Build history of the part. All positions in model axes, mm. Face numbers are marked on the shaded views. Round coordinates to 2 decimals unless told otherwise and drop trailing zeros. Write each loop counter-clockwise with the first axis right and the second up, starting at its lowest first coordinate (ties: lowest second). Pieces come first, ordered by that corner, then holes. Notation, with made-up numbers: (-1.75, 29.5) - (9.25, 29.5) arc R16 ccw to (9.25, 58.5) - close; hole circle Ø9 at (-28.5, 74). An arc over 180 degrees is marked (long way). One line per question, with ' | ' between items.
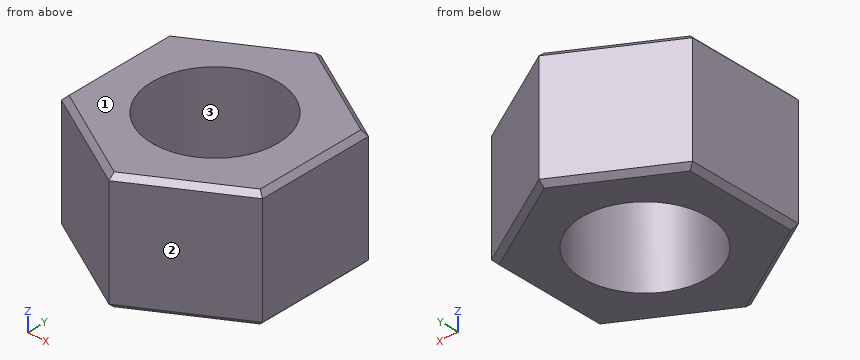
from build123d import *

# Parameters (mm, degrees)
PAD_DEPTH    = 4.7
SKETCH001_R  = 2.5
POCKET_DEPTH = 4.7
CHAMFER_SIZE = 0.2


with BuildPart() as part:
    # Sketch → Pad (new body)
    with BuildSketch(Plane.XY):
        Polygon((-38.60959, 29.262009), (-38.60959, 33.880811), (-42.60959, 36.190212), (-46.60959, 33.880811), (-46.60959, 29.262009), (-42.60959, 26.952608), align=None)
    extrude(amount=PAD_DEPTH)

    # Sketch001 → Pocket (cut)
    with BuildSketch(Plane.XY.offset(4.7)):
        with Locations((-42.60959, 31.57141)):
            Circle(SKETCH001_R)
    extrude(amount=-POCKET_DEPTH, mode=Mode.SUBTRACT)

    # Chamfer
    chamfer_edges = [part.edges().sort_by_distance(p)[0] for p in [
        (-40.60959, 28.107309, 4.7),
        (-38.60959, 31.57141, 4.7),
        (-40.60959, 35.035512, 4.7),
        (-44.60959, 35.035512, 4.7),
        (-46.60959, 31.57141, 4.7),
        (-44.60959, 28.107309, 4.7),
        (-44.60959, 28.107309, 0),
        (-46.60959, 31.57141, 0),
        (-44.60959, 35.035512, 0),
        (-40.60959, 35.035512, 0),
        (-38.60959, 31.57141, 0),
        (-40.60959, 28.107309, 0),
    ]]
    chamfer(chamfer_edges, length=CHAMFER_SIZE)


solid = part.part
Q1. Saw through at B-B, the plane x = -42.25. List the corners of the cut face in (y, z), then the cut area to 3 significant figures.
Found:
outline: (27.16, 0.2) - (27.39, 0) - (29.1, 0) - (29.1, 4.7) - (27.39, 4.7) - (27.16, 4.5) - close; (34.05, 0) - (35.75, 0) - (35.98, 0.2) - (35.98, 4.5) - (35.75, 4.7) - (34.05, 4.7) - close | area: 18.1 mm^2
Q2. Saw through at D-D, the plane z = 2.7. List the corners of the cut face in (x, y).
Found:
outline: (-46.61, 29.26) - (-42.61, 26.95) - (-38.61, 29.26) - (-38.61, 33.88) - (-42.61, 36.19) - (-46.61, 33.88) - close; hole circle Ø5 at (-42.61, 31.57)
Q3. Saw through at A-A, the plane y = 33.25. List the corners of the cut face in (x, z).
Found:
outline: (-46.61, 0.2) - (-46.41, 0) - (-44.46, 0) - (-44.46, 4.7) - (-46.41, 4.7) - (-46.61, 4.5) - close; (-40.76, 0) - (-38.81, 0) - (-38.61, 0.2) - (-38.61, 4.5) - (-38.81, 4.7) - (-40.76, 4.7) - close
Q4. Drop a flat-ended pin along its axis: pin 1 (1 mm diameter, centred on x = -44.5, z = 1, fed in from +Y). Give the stop position or say it passes through.
Found:
pin 1: y = 35.39
Q5. Drill centre lines: L1, parallel to X at y = 31.5, z = 4.4; L2, parallel to Y at x = -42, z = 0.8; L3, parallel to X at y = 31, z = 3.9. Where is each one in solid material? Low to high. Write a range as from..to.
Found:
L1: -46.61..-45.11, -40.11..-38.61 | L2: 27.3..29.15, 34..35.84 | L3: -46.61..-45.04, -40.18..-38.61
Q6. Saw through at C-C, the plane y = 28.75. List the corners of the cut face in (x, z).
Found:
outline: (-45.72, 0.2) - (-45.32, 0) - (-39.9, 0) - (-39.5, 0.2) - (-39.5, 4.5) - (-39.9, 4.7) - (-45.32, 4.7) - (-45.72, 4.5) - close
Q7. Pull direction X, two halves, no side cores. Call the marked faces 1, 2 and 3: +X half, -X half, draft (parallel to the pull), parting line (faces both ways), or undercut.
Found:
face 1: draft | face 2: +X half | face 3: undercut
